Can you work these out from the drawing? Everything is in mm from the part's minimum corner. Give positions to 0.01 mm unless a question says otherwise; leave off trailing zeros. Loops run counter-clockwise (first coordinate to the right, second up) from the corner with the lowest first, then second, coordinate; pieces in that order, holes last. Notation, with made-up numbers: (-3, 88.5) - (12, 88.5) arc R11 ccw to (12, 100.5) - close; hole circle Ø3 at (-36, 70). An arc over 180 degrees is marked (long way). Answer in a Markdown table with one row per item. Add a question column.
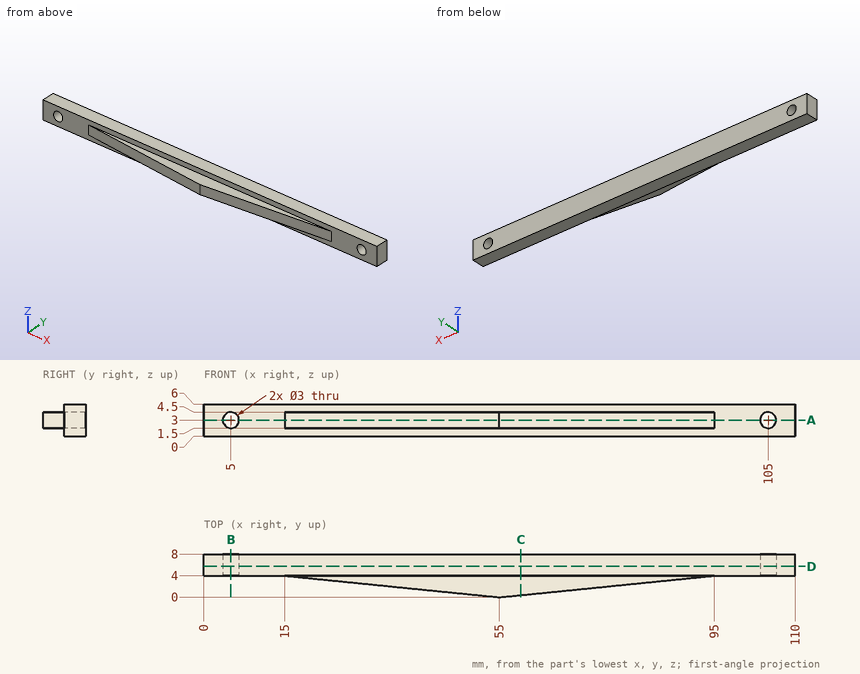
(1) Please list where these lines run through material, in increasing order: line 1 (Z direction, x = 5, y = 5.15); line 2 (X direction, y = 6.25, z = 1.8); line 3 (Y direction, x = 14, z = 3).
(2) For pin 1 Ø2 at (x, y) = (65.5, 1.5) entering from +Z; pin 2 Ø3 at (x, z) = (78.5, 1.5) entering from -Y; pin 3 Ø2 at (x, z) = (73.5, 2) entering from -Y; pin 4 Ø1.8 at (x, z) = (105, 3) entering from -Y, each with a flat end and sliding along its axis, tell me the tip position at first contact or that it passes through.
(3) I want a section at C-C on x = 59. Please give me the cut outline in (y, z).
(4) I want a section at D-D on y = 5.75. Please give me the cut outline in (x, z).
(5) I want a section at A-A on z = 3. Please give me the cut outline in (x, y), then the cut area to 3 significant figures.
(6) I want a section at B-B on x = 5. Please give me the cut outline in (y, z), then the cut area to 3 significant figures.
Reported:
| question | item | result |
|---|---|---|
| 1 | line 1 | 0 to 1.5, 4.5 to 6 |
| 1 | line 2 | 0 to 4.1, 5.9 to 104.1, 105.9 to 110 |
| 1 | line 3 | 4 to 8 |
| 2 | pin 1 | z = 4.5 |
| 2 | pin 2 | y = 2.2 |
| 2 | pin 3 | y = 1.75 |
| 2 | pin 4 | through |
| 3 | outline | (0.4, 1.5) - (4, 1.5) - (4, 0) - (8, 0) - (8, 6) - (4, 6) - (4, 4.5) - (0.4, 4.5) - close |
| 4 | outline | (0, 0) - (110, 0) - (110, 6) - (0, 6) - close; hole circle Ø3 at (5, 3); hole circle Ø3 at (105, 3) |
| 5 | outline | (0, 4) - (3.5, 4) - (3.5, 8) - (0, 8) - close; (6.5, 4) - (15, 4) - (55, 0) - (95, 4) - (103.5, 4) - (103.5, 8) - (6.5, 8) - close; (106.5, 4) - (110, 4) - (110, 8) - (106.5, 8) - close |
| 5 | area | 576 mm² |
| 6 | outline | (4, 0) - (8, 0) - (8, 1.5) - (4, 1.5) - close; (4, 4.5) - (8, 4.5) - (8, 6) - (4, 6) - close |
| 6 | area | 12.0 mm² |
